Here's how the part is built. I have some questions about the finished solid (model axes, mm). Face numbers are marked on the shaded views. A direction names the side the tool comes from. Round coordinates to 2 decimals unless told otherwise and drop trailing zeros. Loops run counter-clockwise (first coordinate to the right, second up) from the corner with the lowest first, then second, coordinate; pieces in that order, holes last. Notation, with made-up numbers: M 1,19 L 13,19 A19 ccw 13,39 Z; hole C -18.5,22.5 d1. An arc over 180 degrees is marked long. Use a Markdown table: item, result.
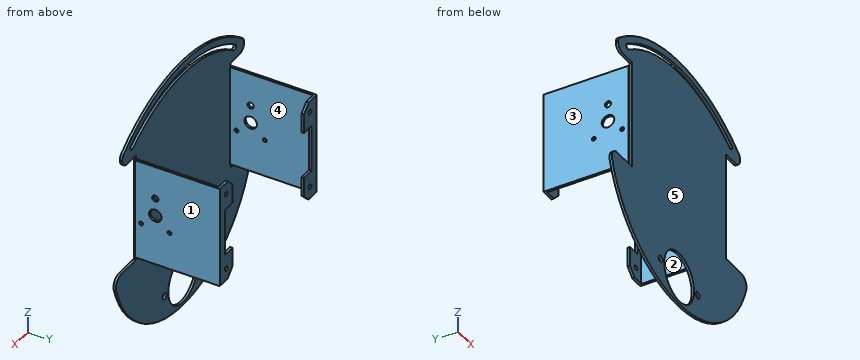
from build123d import *

# Parameters (mm, degrees)
SKETCH_1_R               = 16
EXTRUDE_1_DEPTH          = 1.5
EXTRUDE_START            = 1.5
EXTRUDE_2_DEPTH          = 53.5
SKETCH_5_R               = 4
CUT_EXTRUDE_1_DEPTH      = 54
CUT_EXTRUDE_1_DEPTH_BACK = 73.423245178
EXTRUDE_START_2          = 55.5
EXTRUDE_3_DEPTH          = 1.5
CUT_EXTRUDE_START        = 50
SKETCH_9_R               = 1.5
CUT_EXTRUDE_2_DEPTH      = 6.5
SKETCH_11_R              = 2.05
CUT_EXTRUDE_3_DEPTH      = 2.5
CHAMFER_1_SIZE           = 5
SKETCH_12_R              = 2
SKETCH_12_R_2            = 1.25
CUT_EXTRUDE_4_DEPTH      = 73.423245178
CUT_EXTRUDE_4_DEPTH_BACK = 73.423245178
CUT_EXTRUDE_5_DEPTH      = 10
FILLET_1_R               = 1.6


with BuildPart() as part:
    # Эскиз1 → Бобышка-Вытянуть1 (new body)
    with BuildSketch(Plane(origin=(0, 0, 0), x_dir=(1, 0, 0), z_dir=(0, 1, 0))):
        with BuildLine():
            Line((-50.6, 34.95), (-50.6, 0))
            Line((-50.6, 0), (-50.6, -34.95))
            Line((-50.6, -34.95), (-56.797799253, -34.95))
            Line((-56.797799253, -34.95), (-60.588262065, -34.95))
            ThreePointArc((-60.588262065, -34.95), (-65.306481849, -38.29518821), (-63.711368357, -43.854639175))
            ThreePointArc((-63.711368357, -43.854639175), (0, -66.2), (63.711368357, -43.854639175))
            ThreePointArc((63.711368357, -43.854639175), (65.306481849, -38.29518821), (60.588262065, -34.95))
            Line((60.588262065, -34.95), (50.6, -34.95))
            Line((50.6, -34.95), (50.6, 0))
            Line((50.6, 0), (50.6, 34.95))
            Line((50.6, 34.95), (66.052990091, 34.95))
            Line((66.052990091, 34.95), (66.314478057, 34.95))
            Line((66.314478057, 34.95), (66.423245178, 34.95))
            ThreePointArc((66.423245178, 34.95), (71.249879914, 37.385789411), (72.157626057, 42.715467626))
            ThreePointArc((72.157626057, 42.715467626), (0, 96), (-72.157626057, 42.715467626))
            ThreePointArc((-72.157626057, 42.715467626), (-71.249879914, 37.385789411), (-66.423245178, 34.95))
            Line((-66.423245178, 34.95), (-50.6, 34.95))
        make_face()
        with Locations((0, 78)):
            Circle(SKETCH_1_R, mode=Mode.SUBTRACT)
        with BuildLine():
            Line((-50.6, 34.95), (-50.6, 0))
            Line((-50.6, 0), (-50.6, -34.95))
            Line((-50.6, -34.95), (-56.797799253, -34.95))
            Line((-56.797799253, -34.95), (-60.588262065, -34.95))
            ThreePointArc((-60.588262065, -34.95), (-65.306481849, -38.29518821), (-63.711368357, -43.854639175))
            ThreePointArc((-63.711368357, -43.854639175), (0, -66.2), (63.711368357, -43.854639175))
            ThreePointArc((63.711368357, -43.854639175), (65.306481849, -38.29518821), (60.588262065, -34.95))
            Line((60.588262065, -34.95), (50.6, -34.95))
            Line((50.6, -34.95), (50.6, 0))
            Line((50.6, 0), (50.6, 34.95))
            Line((50.6, 34.95), (66.052990091, 34.95))
            Line((66.052990091, 34.95), (66.314478057, 34.95))
            Line((66.314478057, 34.95), (66.423245178, 34.95))
            ThreePointArc((66.423245178, 34.95), (71.249879914, 37.385789411), (72.157626057, 42.715467626))
            ThreePointArc((72.157626057, 42.715467626), (0, 96), (-72.157626057, 42.715467626))
            ThreePointArc((-72.157626057, 42.715467626), (-71.249879914, 37.385789411), (-66.423245178, 34.95))
            Line((-66.423245178, 34.95), (-50.6, 34.95))
        make_face()
        with Locations((0, 78)):
            Circle(SKETCH_1_R, mode=Mode.SUBTRACT)
        with BuildLine():
            Line((-50.6, 34.95), (-50.6, 0))
            Line((-50.6, 0), (-50.6, -34.95))
            Line((-50.6, -34.95), (-56.797799253, -34.95))
            Line((-56.797799253, -34.95), (-60.588262065, -34.95))
            ThreePointArc((-60.588262065, -34.95), (-65.306481849, -38.29518821), (-63.711368357, -43.854639175))
            ThreePointArc((-63.711368357, -43.854639175), (0, -66.2), (63.711368357, -43.854639175))
            ThreePointArc((63.711368357, -43.854639175), (65.306481849, -38.29518821), (60.588262065, -34.95))
            Line((60.588262065, -34.95), (50.6, -34.95))
            Line((50.6, -34.95), (50.6, 0))
            Line((50.6, 0), (50.6, 34.95))
            Line((50.6, 34.95), (66.052990091, 34.95))
            Line((66.052990091, 34.95), (66.314478057, 34.95))
            Line((66.314478057, 34.95), (66.423245178, 34.95))
            ThreePointArc((66.423245178, 34.95), (71.249879914, 37.385789411), (72.157626057, 42.715467626))
            ThreePointArc((72.157626057, 42.715467626), (0, 96), (-72.157626057, 42.715467626))
            ThreePointArc((-72.157626057, 42.715467626), (-71.249879914, 37.385789411), (-66.423245178, 34.95))
            Line((-66.423245178, 34.95), (-50.6, 34.95))
        make_face()
        with Locations((0, 78)):
            Circle(SKETCH_1_R, mode=Mode.SUBTRACT)
    extrude(amount=EXTRUDE_1_DEPTH)

    # Эскиз3 → Бобышка-Вытянуть2 (add)
    with BuildSketch(Plane(origin=(0, 0, 0), x_dir=(1, 0, 0), z_dir=(0, 1, 0)).offset(EXTRUDE_START)):
        Polygon((-52, 0), (-52, 32.5), (-50.5, 32.5), (-50.5, -32.5), (-52, -32.5), align=None)
        Polygon((52, -32.5), (52, 0), (52, 32.5), (50.5, 32.5), (50.5, -32.5), align=None)
    extrude(amount=EXTRUDE_2_DEPTH)

    # Эскиз5 → Вырез-Вытянуть1 (cut, two sides)
    with BuildSketch(Plane(origin=(0, 0, 0), x_dir=(0, 0, -1), z_dir=(1, 0, 0))) as cut_extrude_1_sk:
        with Locations((0, 14.5)):
            Circle(SKETCH_5_R)
    extrude(amount=CUT_EXTRUDE_1_DEPTH, mode=Mode.SUBTRACT)
    extrude(cut_extrude_1_sk.sketch, amount=-CUT_EXTRUDE_1_DEPTH_BACK, mode=Mode.SUBTRACT)

    # Эскиз6 → Бобышка-Вытянуть3 (add)
    with BuildSketch(Plane(origin=(0, 0, 0), x_dir=(1, 0, 0), z_dir=(0, 1, 0)).offset(EXTRUDE_START_2)):
        Polygon((-52, 32.5), (-52, 0), (-52, -32.5), (-38.5, -32.5), (-38.5, -15), (-46.5, -15), (-46.5, 0), (-46.5, 15), (-38.5, 15), (-38.5, 32.5), align=None)
        Polygon((46.5, 0), (46.5, -15), (38.5, -15), (38.5, -32.5), (52, -32.5), (52, 0), (52, 32.5), (38.5, 32.5), (38.5, 15), (46.5, 15), align=None)
    extrude(amount=-EXTRUDE_3_DEPTH)

    # Эскиз9 → Вырез-Вытянуть2 (cut, through all)
    with BuildSketch(Plane(origin=(0, 0, 0), x_dir=(1, 0, 0), z_dir=(0, 1, 0)).offset(CUT_EXTRUDE_START)):
        with Locations((-45, 25)):
            Circle(SKETCH_9_R)
        with Locations((-45, -25)):
            Circle(SKETCH_9_R)
        with Locations((45, -25)):
            Circle(SKETCH_9_R)
        with Locations((45, 25)):
            Circle(SKETCH_9_R)
    extrude(amount=CUT_EXTRUDE_2_DEPTH, mode=Mode.SUBTRACT)

    # Эскиз11 → Вырез-Вытянуть3 (cut, through all)
    with BuildSketch(Plane(origin=(0, 1.5, 0), x_dir=(1, 0, 0), z_dir=(0, 1, 0))):
        with Locations((20, 78)):
            Circle(SKETCH_11_R)
        with Locations((-20, 78)):
            Circle(SKETCH_11_R)
    extrude(amount=-CUT_EXTRUDE_3_DEPTH, mode=Mode.SUBTRACT)

    # Фаска1
    chamfer_1_edges = [part.edges().sort_by_distance(p)[0] for p in [
        (38.5, 54.75, -32.5),
        (38.5, 54.75, 32.5),
        (-38.5, 54.75, 32.5),
        (-38.5, 54.75, -32.5),
    ]]
    chamfer(chamfer_1_edges, length=CHAMFER_1_SIZE)

    # Эскиз12 → Вырез-Вытянуть4 (cut, two sides)
    with BuildSketch(Plane(origin=(0, 0, 0), x_dir=(0, 0, -1), z_dir=(1, 0, 0))) as cut_extrude_4_sk:
        with Locations((-11.4, 14.5)):
            Circle(SKETCH_12_R)
        with Locations((8.5, 23.5)):
            Circle(SKETCH_12_R_2)
        with Locations((8.5, 5.5)):
            Circle(SKETCH_12_R_2)
    extrude(amount=CUT_EXTRUDE_4_DEPTH, mode=Mode.SUBTRACT)
    extrude(cut_extrude_4_sk.sketch, amount=-CUT_EXTRUDE_4_DEPTH_BACK, mode=Mode.SUBTRACT)

    # Эскиз13 → Вырез-Вытянуть5 (cut)
    with BuildSketch(Plane(origin=(0, 1.5, 0), x_dir=(1, 0, 0), z_dir=(0, 1, 0))):
        with BuildLine():
            Line((0, -62), (0, -58.6))
            ThreePointArc((0, -58.6), (-29.171204269, -53.979735138), (-55.486927816, -40.571204269))
            Line((-55.486927816, -40.571204269), (-57.485397674, -43.32186205))
            ThreePointArc((-57.485397674, -43.32186205), (-30.22186205, -57.213327294), (0, -62))
        make_face()
        with BuildLine():
            ThreePointArc((55.486927816, -40.571204269), (29.171204269, -53.979735138), (0, -58.6))
            Line((0, -58.6), (0, -62))
            ThreePointArc((0, -62), (30.22186205, -57.213327294), (57.485397674, -43.32186205))
            Line((57.485397674, -43.32186205), (55.486927816, -40.571204269))
        make_face()
    extrude(amount=-CUT_EXTRUDE_5_DEPTH, mode=Mode.SUBTRACT)

    # Скругление1
    fillet_1_edges = [part.edges().sort_by_distance(p)[0] for p in [
        (-55.486927816, 0.75, 40.571204269),
        (55.486927816, 0.75, 40.571204269),
        (57.485397674, 0.75, 43.32186205),
        (-57.485397674, 0.75, 43.32186205),
    ]]
    fillet(fillet_1_edges, radius=FILLET_1_R)


solid = part.part
1. Imagine slicing it at B-B, the plane x = -26. Write out the boundary of the cut face in (y, z), then the cut area to 3 significant figures.
Answer sheet:
| item | result |
|---|---|
| outline | M 0,-91.38 L 1.5,-91.38 L 1.5,54.95 L 0,54.95 Z; M 0,58.48 L 1.5,58.48 L 1.5,62.83 L 0,62.83 Z |
| area | 226 mm2 |
2. I need wall thicknesses on probe 1 along Z at (x, y) = (51.1, 23.5); probe 2 along Z at (x, y) = (-45, 54.5); probe 3 along Y at (x, z) = (50, 11). Which ranges of each line are inside material? Lowest first, please. Write a range as from..to.
Answer sheet:
| item | result |
|---|---|
| probe 1 | -32.5..-9.75, -7.25..32.5 |
| probe 2 | -32.5..-26.5, -23.5..-15, 15..23.5, 26.5..32.5 |
| probe 3 | 0..1.5, 54..55.5 |
3. We'd pull the mould along X, two halves only. Please class the marked faces 3, 4 and 5: +X half, -X half, draft (parallel to the pull), parting line (faces both ways), or undercut.
Answer sheet:
| item | result |
|---|---|
| face 3 | -X half |
| face 4 | undercut |
| face 5 | draft |
4. Imagine slicing it at D-D, the plane x = 9.5. Write out the boundary of the cut face in (y, z).
Answer sheet:
| item | result |
|---|---|
| outline | M 0,-95.4 L 1.5,-95.4 L 1.5,-90.87 L 0,-90.87 Z; M 0,-65.13 L 1.5,-65.13 L 1.5,58.12 L 0,58.12 Z; M 0,61.54 L 1.5,61.54 L 1.5,65.76 L 0,65.76 Z |
5. For pin 1 Ø1.2 at (x, y) = (41.5, 55) entering from +Z; pin 2 Ø2.5 at (x, y) = (-49.5, 17) entering from -Z; pin 3 Ø9.5 at (x, z) = (-46.5, 9) entering from -Y; pin 4 Ø2.5 at (y, z) = (14.5, 11.4) entering from -X (1 decimal), each with a flat end and sliding along its axis, tell me the tip position at first contact or that it passes through.
Answer sheet:
| item | result |
|---|---|
| pin 1 | z = 31.1 |
| pin 2 | z = -32.5 |
| pin 3 | y = 0 |
| pin 4 | through |
6. Imagine slicing it at C-C, the plane z = 17.5. Write out the boundary of the cut face in (x, y).
Answer sheet:
| item | result |
|---|---|
| outline | M -52,1.5 L -50.6,1.5 L -50.6,0 L 50.6,0 L 50.6,1.5 L 52,1.5 L 52,55.5 L 38.5,55.5 L 38.5,54 L 50.5,54 L 50.5,1.5 L -50.5,1.5 L -50.5,54 L -38.5,54 L -38.5,55.5 L -52,55.5 Z |
7. Which directions (+Z, -Z, +X, -X, +Y, -Y) give clear straight access to the entire face, cutting with the end or side of a thin tool? Please do the marked faces 1 and 2.
Answer sheet:
| item | result |
|---|---|
| face 1 | +Z, -Z, +X, +Y, -Y |
| face 2 | +Z, -Z |
8. Imagine slicing it at A-A, the plane y = 30. Write out the boundary of the cut face in (x, z).
Answer sheet:
| item | result |
|---|---|
| outline | M -52,-32.5 L -50.5,-32.5 L -50.5,32.5 L -52,32.5 Z; M 50.5,-32.5 L 52,-32.5 L 52,32.5 L 50.5,32.5 Z |
